Here's how the part is built. I have some questions about the finished solid (model axes, mm). A direction names the side the tool comes from. Coordinates: 2 decimals unless noted, no trailing zeros. Write each loop counter-clockwise with the first axis right and the second up, starting at its lowest first coordinate (ties: lowest second). Pieces come first, ordered by that corner, then holes.
(1) Imagine slicing it at A-A, the plane x = -60. List the corners of the cut face in (y, z) for me, plus the area to 3 significant figures.
(2) Imagine slicing it at D-D, the plane y = 0. State how many separate pieces and enclosed holes the cut face has, plus the area to 3 significant figures.
(3) Please list where these lines run through material, in increasing order: probe 1 along X at (y, z) = (0, -5.75); probe 2 along X at (y, z) = (0, 8.75); probe 3 along Y at (x, z) = (-37.5, 8).
(4) Imagine slicing it at C-C, the plane z = 6.5. List the corners of the cut face in (x, y) for me.
(5) Imagine slicing it at B-B, the plane y = -15. List the corners of the cut face in (x, z) for me, plus the area to 3 significant figures.
(6) Which directions (+Z, -Z, +X, -X, +Y, -Y) give clear straight access to the entire face, cutting with the end or side of a thin tool? Please do faces 5 (the cylindrical face through (59.23, 15.43, -3.36)), 6 (the cylindrical face through (57.047, -14.284, 7.704)).
(7) Thinking about a two-plate mould opening in Y: for faces 1 (the flat face through (-1, 30, 0)), 2 (the cylindrical face through (59.23, 0.43, -3.36)), 3 (the cylindrical face through (-55.61, 0.98, -4.39)), 4 (the flat face through (75, 0, 0)), which applies, released by +Y, released by -Y, zero draft, split by the parting line, or undercut?
(8) For pin 1 Ø7.5 at (x, y) = (62.5, 0) entering from +Z; pin 2 Ø12 at (x, y) = (-15, 0) entering from +Z, each with a flat end and sliding along its axis, tell me the tip position at first contact or that it passes through.
Autodesk Inventor part; units mm, degrees
ref_plane "YZ Plane" through (0, 0, 0) normal (1, 0, 0) x (0, 1, 0)
ref_plane "XZ Plane" through (0, 0, 0) normal (0, 1, 0) x (-1, 0, 0)
ref_plane "XY Plane" through (0, 0, 0) normal (0, 0, 1) x (1, 0, 0)
sketch "Sketch2" plane through (0, 0, 0) normal (0, 0, 1) x (1, 0, 0)
  line L0 (75, -30) -> (-75, -30)
  line L1 (-75, -30) -> (-75, 30)
  line L2 (-75, 30) -> (75, 30)
  line L3 (75, 30) -> (75, -30)
  line L4 (75, -30) -> (-75, 30) construction
  line L5 (-75, -30) -> (75, 30) construction
  point P0 (0, 0)
  dimension "d1" = 150
  dimension "d2" = 60
extrude "Extrusion1" add sketch "Sketch2" along normal mid plane 22
sketch "Sketch3" plane through (0, 0, 11) normal (0, 0, 1) x (1, 0, 0)
  line L0 (75, -30) -> (75, 30)
  point P0 (0, 0)
  point P1 (62.5, 0)
  point P2 (62.5, 15)
  point P3 (62.5, -15)
  point P4 (75, 0)
  dimension "d5" = 12.5
  dimension "d6" = 30
  dimension "d7" = 15
hole "Hole1" at (62.5, 0, 11) at (62.5, 15, 11) at (62.5, -15, 11) direction (0, 0, -1) diameter 6.6 end through all counterbore diameter 11 counterbore depth 6.5
sketch "Sketch4" plane through (0, 0, 11) normal (0, 0, 1) x (1, 0, 0)
  line L0 (-75, 30) -> (-75, -30)
  point P0 (0, 0)
  point P1 (-60, 0)
  point P2 (-37.5, 0)
  point P3 (-15, 0)
  point P4 (-75, 0)
  point P5 (-75, 0)
  dimension "d15" = 15
  dimension "d16" = 22.5
  dimension "d17" = 22.5
hole "Hole2" at (-60, 0, 11) at (-37.5, 0, 11) at (-15, 0, 11) direction (0, 0, -1) diameter 9 end through all counterbore diameter 15 counterbore depth 8.6
chamfer "Chamfer2" distance 2 angle 45 4 edges at (75, 0, 11) (75, 0, -11) (-75, 0, 11) (-75, 0, -11)
properties part number "TL20240901-10320CV-021" material "SS400"
Recorded:
1. outline: (-30, -11) - (-4.5, -11) - (-4.5, 2.4) - (-7.5, 2.4) - (-7.5, 11) - (-30, 11) - close; (4.5, -11) - (30, -11) - (30, 11) - (7.5, 11) - (7.5, 2.4) - (4.5, 2.4) - close
1. area: 1,070 mm2
2. separate pieces: 5
2. enclosed holes: 0
2. area: 2,370 mm2
3. probe 1: x = -75 to -64.5, -55.5 to -42, -33 to -19.5, -10.5 to 59.2, 65.8 to 75
3. probe 2: x = -75 to -67.5, -52.5 to -45, -30 to -22.5, -7.5 to 57, 68 to 75
3. probe 3: y = -30 to -7.5, 7.5 to 30
4. outline: (-75, -30) - (75, -30) - (75, 30) - (-75, 30) - close; hole circle Ø15 at (-60, 0); hole circle Ø15 at (-37.5, 0); hole circle Ø15 at (-15, 0); hole circle Ø11 at (62.5, -15); hole circle Ø11 at (62.5, 0); hole circle Ø11 at (62.5, 15)
5. outline: (-75, -9) - (-73, -11) - (59.2, -11) - (59.2, 4.5) - (57, 4.5) - (57, 11) - (-73, 11) - (-75, 9) - close; (65.8, -11) - (73, -11) - (75, -9) - (75, 9) - (73, 11) - (68, 11) - (68, 4.5) - (65.8, 4.5) - close
5. area: 3,120 mm2
6. face 5: +Z, -Z
6. face 6: +Z
7. face 1: released by +Y
7. face 2: undercut
7. face 3: undercut
7. face 4: zero draft
8. pin 1: stops at z = 4.5
8. pin 2: stops at z = 2.4
